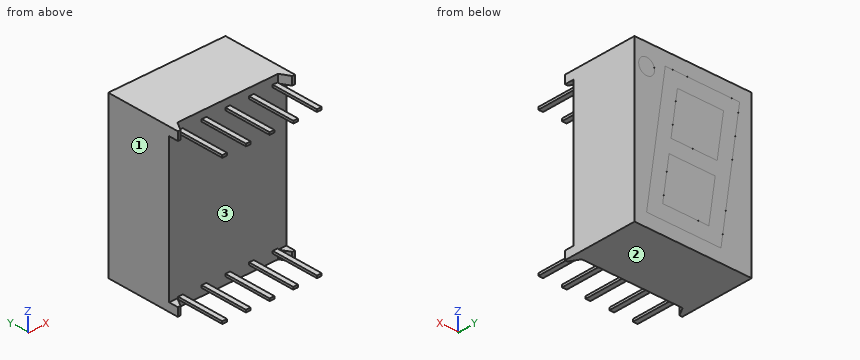
```python
from build123d import *

# Parameters (mm, degrees)
EXTRUDE1_DEPTH          = 6.2865
SKETCH4_R               = 0.85
CUT_EXTRUDE1_DEPTH      = 0.001
CUT_EXTRUDE2_DEPTH      = 14.264244504
CUT_EXTRUDE2_DEPTH_BACK = 14.264244504
SKETCH2_W               = 0.51
SKETCH2_H               = 0.254
EXTRUDE2_DEPTH          = 5.09
LPATTERN1_COUNT         = 3
LPATTERN1_PITCH         = 2.54
LPATTERN1_COL_COUNT     = 3
LPATTERN1_COL_PITCH     = 2.54


with BuildPart() as part:
    # Sketch1 → Extrude1 (new, symmetric)
    with BuildSketch(Plane(origin=(0, 0, 0), x_dir=(0, 0, -1), z_dir=(1, 0, 0))):
        Polygon((-8.51, 0), (8.51, 0), (8.51, -8), (7.62, -8), (7.62, -7), (-7.62, -7), (-7.62, -8), (-8.51, -8), align=None)
    extrude(amount=EXTRUDE1_DEPTH, both=True)

    # Sketch4 → Cut-Extrude1 (cut)
    # profile 1 of 2: a face of its own
    with BuildSketch(Plane(origin=(0, 0, 0), x_dir=(-1, 0, 0), z_dir=(0, 1, 0))):
        with Locations(Location((-4.988064246, 6.26, 0), (0, 0, 90))):
            Circle(SKETCH4_R)
    # profile 2 of 2: a face of its own
    with BuildSketch(Plane(origin=(0, 0, 0), x_dir=(-1, 0, 0), z_dir=(0, 1, 0))):
        Polygon((4.988064246, 7.11), (2.989573577, -7.11), (-4.988064246, -7.11), (-2.989573577, 7.11), align=None)
        Polygon((-1.68564347, 5.61), (3.262511635, 5.61), (2.579483179, 0.75), (-2.368671927, 0.75), align=None, mode=Mode.SUBTRACT)
        Polygon((-3.262511635, -5.61), (-2.579483179, -0.75), (2.368671927, -0.75), (1.68564347, -5.61), align=None, mode=Mode.SUBTRACT)
    extrude(amount=-CUT_EXTRUDE1_DEPTH, mode=Mode.SUBTRACT)

    # Sketch5 → Cut-Extrude2 (cut, two sides: drawn at the far end of the back side and taken through both)
    with BuildSketch(Plane.XY.offset(-CUT_EXTRUDE2_DEPTH_BACK)):
        Polygon((-5.9865, -8), (-5.409149731, -7), (5.409149731, -7), (5.9865, -8), align=None)
    extrude(amount=CUT_EXTRUDE2_DEPTH + CUT_EXTRUDE2_DEPTH_BACK, mode=Mode.SUBTRACT)

    # Sketch2 → Extrude2 (add)
    with BuildSketch(Plane.XZ.offset(7)):
        with Locations((0, 7.62)):
            Rectangle(SKETCH2_W, SKETCH2_H)
        with Locations((0, -7.62)):
            Rectangle(SKETCH2_W, SKETCH2_H)
    extrude2 = extrude(amount=EXTRUDE2_DEPTH)

    # LPattern1: Extrude2 ×3
    with Locations(*[(i * LPATTERN1_PITCH, 0, 0) for i in range(1, LPATTERN1_COUNT)]):
        add(extrude2)

    # LPattern1 col: Extrude2 ×3
    with Locations(*[(-i * LPATTERN1_COL_PITCH, 0, 0) for i in range(1, LPATTERN1_COL_COUNT)]):
        add(extrude2)


solid = part.part
```
Build history of the part. All positions in model axes, mm. Face numbers are marked on the shaded views. Round coordinates to 2 decimals unless told otherwise and drop trailing zeros.
Item 1: Drill centre lines: line 1 along Z through (x, y) = (-2.5, -10.25); line 2 along Y through (x, z) = (-5, -0.75). Where is each one in solid material? Low to high.
Item 2: Two-plate mould, pull along Z, no slides. Class the marked faces 1, 2 and 3: released by +Z, released by -Z, zero draft, split by the parting line, or undercut.
Item 3: Pin check, flat tips, straight feed: P1, Ø6, axis at y = -8, z = -6, coming from the -X side; P2, Ø5, axis at x = 4.5, z = -1.5, coming from the -Y side; P3, Ø1.5, axis at x = 1.5, y = -9, coming from the -Z side. Stop position of each tip, or through.
Worked answers:
1. line 1: z = -7.75 to -7.49, 7.49 to 7.75
1. line 2: y = -7 to 0
2. face 1: zero draft
2. face 2: released by -Z
2. face 3: undercut
3. P1: stops at x = -6.29
3. P2: stops at y = -7
3. P3: passes through
